from build123d import *
from OCP.BRepFilletAPI import BRepFilletAPI_MakeChamfer

# Parameters (mm, degrees)
BOSS_EXTRUDE1_DEPTH     = 16.399996177
CUT_EXTRUDE1_DEPTH      = 32.345970628
CUT_EXTRUDE3_DEPTH      = 30.483891782
CUT_EXTRUDE3_DEPTH_BACK = 30.483891782
SKETCH4_R               = 4.2
BOSS_EXTRUDE2_START     = -14.4
BOSS_EXTRUDE2_DEPTH     = 14.4
SKETCH6_W               = 16.399996177
SKETCH6_H               = 5
CUT_EXTRUDE4_DEPTH      = 10
FILLET1_R               = 12
CHAMFER1_SIZE           = 0.5
CHAMFER2_SIZE           = 0.5
CHAMFER2_SIZE2          = 1.366025404


with BuildPart() as part:
    # Sketch1 → Boss-Extrude1 (new body)
    with BuildSketch(Plane.XY.offset(16.399996177)):
        with BuildLine():
            Line((7.2, 0), (22.5, 0))
            Line((22.5, 0), (22.5, 14.4))
            Line((22.5, 14.4), (7.2, 14.4))
            ThreePointArc((7.2, 14.4), (0, 7.2), (7.2, 0))
        make_face()
    extrude(amount=-BOSS_EXTRUDE1_DEPTH)

    # Sketch2 → Cut-Extrude1 (cut, through all)
    with BuildSketch(Plane(origin=(0, 0, 0), x_dir=(-1, 0, 0), z_dir=(0, 0, -1))):
        with BuildLine():
            Line((-22.5, 9.7), (-22.5, 4.7))
            Line((-22.5, 4.7), (-10.532688106, 4.7))
            ThreePointArc((-10.532688106, 4.7), (-2.9577807, 7.2), (-10.532688106, 9.7))
            Line((-10.532688106, 9.7), (-22.5, 9.7))
        make_face()
    extrude(amount=-CUT_EXTRUDE1_DEPTH, mode=Mode.SUBTRACT)

    # Sketch4 → Cut-Extrude3 (cut, two sides: drawn at the far end of the back side and taken through both)
    with BuildSketch(Plane.XZ.offset(-9.7).offset(-CUT_EXTRUDE3_DEPTH_BACK)):
        with Locations((17, 8.2)):
            Circle(SKETCH4_R)
    extrude(amount=CUT_EXTRUDE3_DEPTH + CUT_EXTRUDE3_DEPTH_BACK, mode=Mode.SUBTRACT)

    # Sketch5 → Boss-Extrude2 (add)
    with BuildSketch(Plane(origin=(0, 14.4, 0), x_dir=(1, 0, 0), z_dir=(0, 1, 0)).offset(BOSS_EXTRUDE2_START)):
        Polygon((22.5, 0), (22.5, -16.399996177), (27.234271104, -8.199998088), align=None)
    boss_extrude2 = extrude(amount=BOSS_EXTRUDE2_DEPTH)

    # Mirror3: Boss-Extrude2 across plane
    add(boss_extrude2.mirror(Plane(origin=(0, 7.2, 0), x_dir=(0, 0, 1), z_dir=(0, -1, 0))))

    # Sketch6 → Cut-Extrude4 (cut)
    with BuildSketch(Plane.ZY.offset(-22.5)):
        with Locations((8.199998089, 7.2)):
            Rectangle(SKETCH6_W, SKETCH6_H)
    extrude(amount=-CUT_EXTRUDE4_DEPTH, mode=Mode.SUBTRACT)

    # Fillet1
    fillet1_edges = [part.edges().sort_by_distance(p)[0] for p in [
        (27.234271104, 2.35, 8.199998088),
        (27.234271104, 12.05, 8.199998088),
    ]]
    fillet(fillet1_edges, radius=FILLET1_R)

    # Chamfer1
    chamfer1_edges = [part.edges().sort_by_distance(p)[0] for p in [
        (2.9577807, 7.2, 16.399996177),
    ]]
    chamfer(chamfer1_edges, length=CHAMFER1_SIZE)

    # Chamfer2: one chamfer whose edges measure the first distance from different faces: ONE call of the kernel's chamfer builder (chamfer() names one face for all edges)
    chamfer2_edges_1 = [part.edges().sort_by_distance(p)[0] for p in [
        (22.5, 12.05, 16.399996177),
    ]]
    chamfer2_side_1 = [part.faces().sort_by_distance(p)[0] for p in [
        (23.135084744, 12.05, 15.299997133),
    ]]
    chamfer2_edges_2 = [part.edges().sort_by_distance(p)[0] for p in [
        (22.5, 2.35, 16.399996177),
    ]]
    chamfer2_side_2 = [part.faces().sort_by_distance(p)[0] for p in [
        (23.135084744, 2.35, 15.299997133),
    ]]
    chamfer2_edges_3 = [part.edges().sort_by_distance(p)[0] for p in [
        (14.85, 0, 16.399996177),
        (0, 7.2, 16.399996177),
        (14.85, 14.4, 16.399996177),
        (16.818865224, 9.7, 16.399996177),
        (16.818865224, 4.7, 16.399996177),
    ]]
    chamfer2 = BRepFilletAPI_MakeChamfer(part.part.solid().wrapped)
    for e in chamfer2_edges_1:
        chamfer2.Add(CHAMFER2_SIZE, CHAMFER2_SIZE2, e.wrapped, chamfer2_side_1[0].wrapped)  # the first distance lies on this face
    for e in chamfer2_edges_2:
        chamfer2.Add(CHAMFER2_SIZE, CHAMFER2_SIZE2, e.wrapped, chamfer2_side_2[0].wrapped)  # the first distance lies on this face
    for e in chamfer2_edges_3:
        chamfer2.Add(CHAMFER2_SIZE, e.wrapped)
    add(Compound.cast(chamfer2.Shape()), mode=Mode.REPLACE)


solid = part.part
The listing builds one solid part. Answer for the finished solid, in the listing's coordinates (mm). A direction names the side the tool comes from. Give positions to 0.01 mm unless a question says otherwise; leave off trailing zeros. Write each loop counter-clockwise with the first axis right and the second up, starting at its lowest first coordinate (ties: lowest second). Pieces come first, ordered by that corner, then holes. Notation, with made-up numbers: (42.5, 51) -> (91.5, 51) arc R14 ccw to (91.5, 59) -> close; hole circle Ø7 at (-4.75, 43). An arc over 180 degrees is marked (long way). Use a Markdown table: item, result.
(1) Section D-D, the plane y = 7.2 is taken. Determine the outline of the cut face in (x, z), then the cut area to 3 significant figures.
Return value:
| item | result |
|---|---|
| outline | (0, 0) -> (2.96, 0) -> (2.96, 15.9) -> (2.46, 16.4) -> (0.5, 16.4) -> (0, 15.9) -> close |
| area | 48.3 mm2 |
(2) Determine the mould class of faces 3 (the cylindrical face through (0, 7.36, 8.06)), 4 (the conical face through (2.82, 7.05, 16.04)), 5 (the flat face through (21, 9.7, 6)) for opening direction X: released by +X, released by -X, zero draft, split by the parting line, or undercut.
Return value:
| item | result |
|---|---|
| face 3 | released by -X |
| face 4 | undercut |
| face 5 | zero draft |
(3) Flat-ended cylindrical pins translate along their axes: P1, Ø1.5, axis at y = 9.5, z = 6.5, coming from the +X side; P2, Ø1, axis at x = 4, z = 2, coming from the +Y side; P3, Ø1.5, axis at y = 3.5, z = 5, coming from the +X side. Find the tip coordinate at first contact, or state that the pin passes through.
Return value:
| item | result |
|---|---|
| P1 | x = 25.34 |
| P2 | y = 13.87 |
| P3 | x = 25.13 |
(4) Section B-B, the plane x = 17 is taken. Determine the outline of the cut face in (y, z), then the cut area to 3 significant figures.
Return value:
| item | result |
|---|---|
| outline | (0, 0) -> (4.7, 0) -> (4.7, 4) -> (0, 4) -> close; (0, 12.4) -> (4.7, 12.4) -> (4.7, 15.9) -> (4.2, 16.4) -> (0.5, 16.4) -> (0, 15.9) -> close; (9.7, 0) -> (14.4, 0) -> (14.4, 4) -> (9.7, 4) -> close; (9.7, 12.4) -> (14.4, 12.4) -> (14.4, 15.9) -> (13.9, 16.4) -> (10.2, 16.4) -> (9.7, 15.9) -> close |
| area | 74.7 mm2 |
(5) Section C-C, the plane x = 12.25 is taken. Determine the outline of the cut face in (y, z), then the cut area to 3 significant figures.
Return value:
| item | result |
|---|---|
| outline | (0, 0) -> (4.7, 0) -> (4.7, 15.9) -> (4.2, 16.4) -> (0.5, 16.4) -> (0, 15.9) -> close; (9.7, 0) -> (14.4, 0) -> (14.4, 15.9) -> (13.9, 16.4) -> (10.2, 16.4) -> (9.7, 15.9) -> close |
| area | 154 mm2 |
(6) Find the intervals of material crossed by probe 1 along Y at (x, z) = (19, 14.25); probe 2 along Z at (x, y) = (17, 11.3); probe 3 along X at (y, z) = (12.25, 9.5), in increasing order. Write a range as from..to.
Return value:
| item | result |
|---|---|
| probe 1 | 0..4.7, 9.7..14.4 |
| probe 2 | 0..4, 12.4..16.4 |
| probe 3 | 2.07..13.01, 20.99..25.31 |
(7) Section A-A, the plane z = 8.2 is taken. Determine the outline of the cut face in (x, y), then the cut area to 3 significant figures.
Return value:
| item | result |
|---|---|
| outline | (7.2, 0) -> (12.8, 0) -> (12.8, 4.7) -> (10.53, 4.7) arc R4.2 cw (long way) to (10.53, 9.7) -> (12.8, 9.7) -> (12.8, 14.4) -> (7.2, 14.4) arc R7.2 ccw to start; (21.2, 0) -> (25.38, 0) -> (25.38, 4.7) -> (21.2, 4.7) -> close; (21.2, 9.7) -> (25.38, 9.7) -> (25.38, 14.4) -> (21.2, 14.4) -> close |
| area | 137 mm2 |
(8) For faces 1 (the flat face through (21.4, 4.7, 7.8)), 2 (the flat face through (23.144, 12.017, 1.115)), determine the directions among +Z, -Z, +X, -X, +Y, -Y from which every point of the face is accessible in a straight line to the end or side of a thin tool.
Return value:
| item | result |
|---|---|
| face 1 | +Z, -Z, +X |
| face 2 | -Z, +X, +Y, -Y |
